Read the model definition and answer for the solid it produces. Units are mm, in the model's axes. Face numbers are marked on the shaded views. A direction names the side the tool comes from. Give positions to 0.01 mm unless a question says otherwise; leave off trailing zeros. Write each loop counter-clockwise with the first axis right and the second up, starting at its lowest first coordinate (ties: lowest second). Pieces come first, ordered by that corner, then holes. Notation, with made-up numbers: (35.25, 63.5) - (71.25, 63.5) arc R28 ccw to (71.25, 92.5) - close; hole circle Ø8 at (14.25, -26.5). An arc over 180 degrees is marked (long way). Use CSV: the item, a comma, the result in double quotes. Start each with the question number.
from build123d import *

# Parameters (mm, degrees)
SKETCH_1_W          = 136
SKETCH_1_H          = 104
EXTRUDE_1_DEPTH     = 42
SKETCH_2_W          = 116
SKETCH_2_H          = 84
CUT_EXTRUDE_1_DEPTH = 36
SKETCH_6_R          = 2.2
CUT_EXTRUDE_5_DEPTH = 136
SKETCH_7_R          = 2.2
CUT_EXTRUDE_6_DEPTH = 104


with BuildPart() as part:
    # 草图1 → 凸台-拉伸1 (new body)
    with BuildSketch(Plane(origin=(0, 0, 0), x_dir=(1, 0, 0), z_dir=(0, 1, 0))):
        Rectangle(SKETCH_1_W, SKETCH_1_H)
    extrude(amount=EXTRUDE_1_DEPTH)

    # 草图2 → 切除-拉伸1 (cut)
    with BuildSketch(Plane(origin=(0, 42, 0), x_dir=(1, 0, 0), z_dir=(0, 1, 0))):
        Rectangle(SKETCH_2_W, SKETCH_2_H)
    extrude(amount=-CUT_EXTRUDE_1_DEPTH, mode=Mode.SUBTRACT)

    # 草图6 → 切除-拉伸5 (cut)
    with BuildSketch(Plane.ZY.offset(68)):
        with Locations((-26, 21)):
            Circle(SKETCH_6_R)
        with Locations((26, 21)):
            Circle(SKETCH_6_R)
        with Locations((0, 21)):
            Circle(SKETCH_6_R)
    extrude(amount=-CUT_EXTRUDE_5_DEPTH, mode=Mode.SUBTRACT)

    # 草图7 → 切除-拉伸6 (cut)
    with BuildSketch(Plane(origin=(0, 0, -52), x_dir=(-1, 0, 0), z_dir=(0, 0, -1))):
        with Locations((-34, 21)):
            Circle(SKETCH_7_R)
        with Locations((34, 21)):
            Circle(SKETCH_7_R)
        with Locations((0, 21)):
            Circle(SKETCH_7_R)
    extrude(amount=-CUT_EXTRUDE_6_DEPTH, mode=Mode.SUBTRACT)


solid = part.part
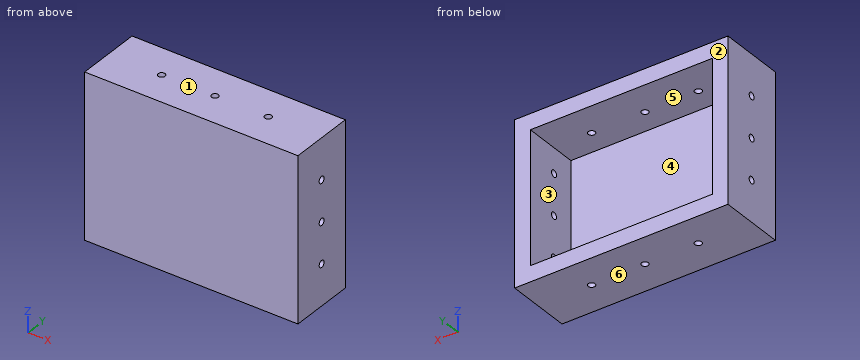
(1) Given P1, Ø4, axis at x = -50, z = -31, coming from the +Y side, flat-ended and moving along its own axis, determine where the tip first touches the part or whether it passes through.
(2) Consider probe 1 along X at (y, z) = (12, 32.5); probe 2 along Y at (x, z) = (63.5, 26); probe 3 along Z at (x, y) = (-1.5, 25.5). Determine where each line is inside the solid, lowest interval first.
(3) The part is cut by section D-D on x = 53. Write down the section's boundary in (y, z).
(4) The part is cut by section A-A on x = 34. Write down the section's boundary in (y, z), plus the area to 3 significant figures.
(5) Which of the six approach directions +Z, -Z, +X, -X, +Y, -Y give full straight-line access (tool end or side, diameter ignored) to the marked faces 5 and 6?
(6) The part is cut by section B-B on y = 39.5. Write down the section's boundary in (x, z).
(7) The part is cut by section C-C on z = 0. Write down the section's boundary in (x, y).
(8) For a pull along Z with two mould halves and no side action, classify the marked faces 1, 2, 3 and 4 as pulls with the +Z half, pulls with the -Z half, needs draft (parallel to the pull), parting line crosses it, or undercut.
Reported:
1,P1,"y = 6"
2,probe 1,"-68 to -58, 58 to 68"
2,probe 2,"0 to 18.8, 23.2 to 42"
2,probe 3,"-52 to -42, 42 to 52"
3,outline,"(0, -52) - (42, -52) - (42, -42) - (6, -42) - (6, 42) - (42, 42) - (42, 52) - (0, 52) - close"
4,outline,"(0, -52) - (18.8, -52) - (18.8, -42) - (6, -42) - (6, 42) - (18.8, 42) - (18.8, 52) - (0, 52) - close; (23.2, -52) - (42, -52) - (42, -42) - (23.2, -42) - close; (23.2, 42) - (42, 42) - (42, 52) - (23.2, 52) - close"
4,area,"1,260 mm²"
5,face 5,"+Y"
5,face 6,"-Z, +X, -X, +Y, -Y"
6,outline,"(-68, -52) - (68, -52) - (68, 52) - (-68, 52) - close; hole (-58, -42) - (58, -42) - (58, 42) - (-58, 42) - close"
7,outline,"(-68, 0) - (68, 0) - (68, 18.8) - (58, 18.8) - (58, 6) - (-58, 6) - (-58, 18.8) - (-68, 18.8) - close; (-68, 23.2) - (-58, 23.2) - (-58, 42) - (-68, 42) - close; (58, 23.2) - (68, 23.2) - (68, 42) - (58, 42) - close"
8,face 1,"pulls with the +Z half"
8,face 2,"needs draft"
8,face 3,"undercut"
8,face 4,"undercut"
